Model file for the job. Use its own axes, mm. Round coordinates to 2 decimals unless told otherwise and drop trailing zeros. Order: outer loops, then holes, each group sorted by start corner. A loop starts at its lowest first (then second) coordinate and runs counter-clockwise, first axis right, second up. Notation, with made-up numbers: (3.5, 1) - (10.5, 1) arc R12 ccw to (10.5, 12) - close; hole circle Ø6 at (3, -2.5). An arc over 180 degrees is marked (long way). Put each result on its own line as item: value. Start each with the question number.
Item 1: Saw through at B-B on z = 23.5. List the corners of the cut face in (x, y).
Item 2: Probe probe 1 along Z at (x, y) = (-42.5, -17.5); probe 2 along Z at (x, y) = (-42, -7.5); probe 3 along X at (y, z) = (-24, 3). List the from-to ranges inside material, lowest first.
Item 3: Saw through at A-A on x = -22. List the corners of the cut face in (y, z).
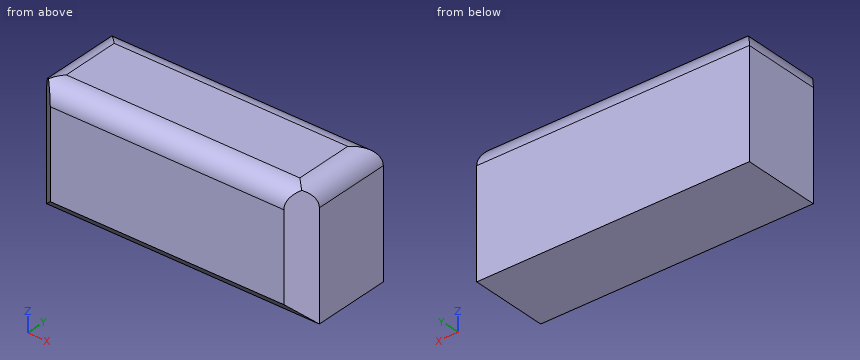
```python
from build123d import *

# Parameters (mm, degrees)
F1_DEPTH    = 25.4
F2_R        = 5.08
F3_T1_DEPTH = 53.8847270698
F3_T3_DEPTH = 97.0179937739


# Not quite as in the source:
# - a fillet or chamfer that OpenCascade refuses, or shapes differently, is made with other operations: its cross-section is extruded or revolved along the edge and cut away or added


with BuildPart() as f1:
    # F0 (on Front) → F1 (new body)
    with BuildSketch(Plane.XZ):
        with BuildLine():
            ThreePointArc((-26.0082527554, 9.7501287237), (-33.751696872, 20.4773638636), (-46.3714562356, 16.5054406347))
            Line((-46.3714562356, 16.5054406347), (-46.3714562356, 2.9948168126))
            ThreePointArc((-46.3714562356, 2.9948168126), (-33.751696872, -0.9771064163), (-26.0082527554, 9.7501287237))
        make_face()
        with BuildLine():
            Line((24.5182383806, 25.2565909177), (-46.3714562356, 25.2565909177))
            Line((-46.3714562356, 25.2565909177), (-46.3714562356, 16.5054406347))
            ThreePointArc((-46.3714562356, 16.5054406347), (-33.751696872, 20.4773638636), (-26.0082527554, 9.7501287237))
            ThreePointArc((-26.0082527554, 9.7501287237), (-33.751696872, -0.9771064163), (-46.3714562356, 2.9948168126))
            Line((-46.3714562356, 2.9948168126), (-46.3714562356, -7.5798369944))
            Line((-46.3714562356, -7.5798369944), (24.5182383806, -7.5798369944))
            Line((24.5182383806, -7.5798369944), (24.5182383806, 25.2565909177))
        make_face()
    extrude(amount=F1_DEPTH)

    # F2
    f2_edges = [f1.edges().sort_by_distance(p)[0] for p in [
        (24.518238, -12.7, 25.256591),
        (-46.371456, -12.7, 25.256591),
        (-10.926609, 0, 25.256591),
        (-10.926609, -25.4, 25.256591),
    ]]
    fillet(f2_edges, radius=F2_R)

    # F3: chamfer of 5.08 on 4 edges, made by hand

    # F3_s2 → F3_t1 (cut)
    with BuildSketch(Plane.XY.offset(-20.6439865733)):
        Polygon((-41.2914562356, -25.4), (-46.3714562356, -20.32), (-46.3714562356, -25.4), align=None)
        Polygon((24.5182383806, -20.32), (19.4382383806, -25.4), (24.5182383806, -25.4), align=None)
    extrude(amount=F3_T1_DEPTH, mode=Mode.SUBTRACT)

    # F3_s4 → F3_t3 (cut)
    with BuildSketch(Plane.YZ.offset(-59.4356058145)):
        Polygon((-20.32, -7.5798369944), (-25.4, -2.4998369944), (-25.4, -7.5798369944), align=None)
    extrude(amount=F3_T3_DEPTH, mode=Mode.SUBTRACT)


solid = f1.part
```
Results found:
1. outline: (-45.13, -21.56) - (-42.53, -24.16) - (20.68, -24.16) - (23.28, -21.56) - (23.28, -1.24) - (-45.13, -1.24) - close
2. probe 1: z = -7.58 to 25.11
2. probe 2: z = -7.58 to 25.21
2. probe 3: x = -42.69 to 20.84
3. outline: (-25.4, -2.5) - (-20.32, -7.58) - (0, -7.58) - (0, 20.18) arc R5.08 ccw to (-5.08, 25.26) - (-20.32, 25.26) arc R5.08 ccw to (-25.4, 20.18) - close
